For this review, take the finished solid that the model builds, in its own axes (mm). Face numbers are marked on the shaded views. A direction names the side the tool comes from. Give positions to 0.01 mm unless a question says otherwise; leave off trailing zeros. Write each loop counter-clockwise with the first axis right and the second up, starting at its lowest first coordinate (ties: lowest second). Pieces come first, ordered by that corner, then holes. Notation, with made-up numbers: M -3.75,-24.75 L 4.25,-24.75 A14 ccw 4.25,-8.75 Z; hole C -36.75,84 d11. An arc over 180 degrees is marked long. Answer as a JSON object with one key per item and string values. Group by question number.
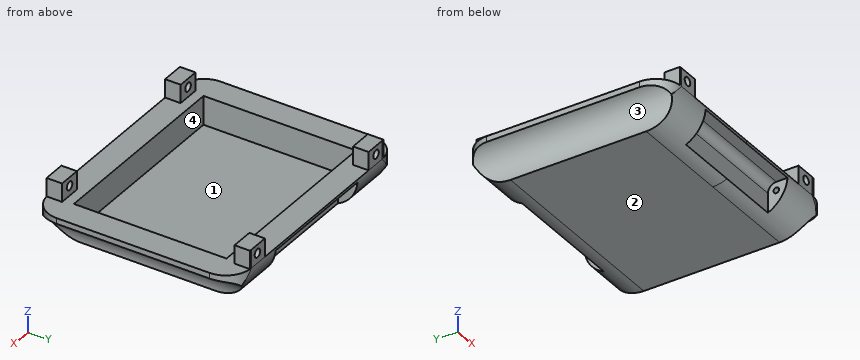
```python
from build123d import *

# Parameters (mm, degrees)
PAD003_DEPTH               = 18
POCKET008_DEPTH            = 22.126
POCKET008_DEPTH_BACK       = 22.126
SKETCH014_W                = 27
SKETCH014_H                = 5.1
POCKET009_DEPTH            = 17.5
POCKET010_DEPTH            = 11.05
SKETCH016_R                = 0.5
POCKET011_DEPTH            = 13.5
SKETCH018_W                = 4
SKETCH018_H                = 3.25
SKETCH018_R                = 0.75
PAD004_DEPTH               = 2.75
SKETCH018_MIRRORED005_2_W  = 4
SKETCH018_MIRRORED005_2_H  = 3.25
SKETCH018_MIRRORED005_2_R  = 0.75
PAD004_MIRRORED005_2_DEPTH = 2.75
SKETCH010_W                = 70
SKETCH010_H                = 70
POCKET013_DEPTH            = 6.001
POCKET013_DEPTH_BACK       = 3.251


with BuildPart() as part:
    # Sketch009 → Pad003 (new body, symmetric)
    with BuildSketch(Plane.XZ):
        with BuildLine():
            Line((-22.125, 0), (22.125, 0))
            Line((22.125, 0), (22.125, -1))
            ThreePointArc((22.125, -1), (19.164351, -2.759027), (18, -6))
            Line((-18, -6), (18, -6))
            ThreePointArc((-18, -6), (-19.164351, -2.759027), (-22.125, -1))
            Line((-22.125, 0), (-22.125, -1))
        make_face()
    extrude(amount=PAD003_DEPTH, both=True)

    # Sketch013 → Pocket008 (cut, two sides)
    with BuildSketch(Plane.YZ) as pocket008_sk:
        with BuildLine():
            ThreePointArc((-18, 0), (-16.242641, -4.242641), (-12, -6))
            Line((-12, -6), (-18, -6))
            Line((-18, 0), (-18, -6))
        make_face()
        with BuildLine():
            ThreePointArc((12, -6), (16.242641, -4.242641), (18, 0))
            Line((18, 0), (18, -6))
            Line((12, -6), (18, -6))
        make_face()
    extrude(amount=-POCKET008_DEPTH, mode=Mode.SUBTRACT)
    extrude(pocket008_sk.sketch, amount=POCKET008_DEPTH_BACK, mode=Mode.SUBTRACT)

    # Sketch014 → Pocket009 (cut, symmetric)
    with BuildSketch(Plane.YZ):
        with Locations((0, -2.55)):
            Rectangle(SKETCH014_W, SKETCH014_H)
    pocket009 = extrude(amount=POCKET009_DEPTH, both=True, mode=Mode.SUBTRACT)

    # Sketch015 → Pocket010 (cut, symmetric)
    with BuildSketch(Plane.YZ):
        with BuildLine():
            Line((16, -0.5), (18, -0.5))
            Line((18, -0.5), (18, -6))
            Line((18, -6), (14.5, -6))
            Line((14.5, -6), (14.5, -2))
            ThreePointArc((16, -0.5), (14.93934, -0.93934), (14.5, -2))
        make_face()
    pocket010 = extrude(amount=POCKET010_DEPTH, both=True, mode=Mode.SUBTRACT)

    # Sketch016 → Pocket011 (cut, symmetric)
    with BuildSketch(Plane.YZ):
        with Locations((16, -2)):
            Circle(SKETCH016_R)
    pocket011 = extrude(amount=POCKET011_DEPTH, both=True, mode=Mode.SUBTRACT)

    # Mirrored004: Pocket009, Pocket010, Pocket011 across Sketch014 V_Axis
    add(pocket009.mirror(Plane(origin=(0, 0, 0), x_dir=(1, 0, 0), z_dir=(0, 1, 0))), mode=Mode.SUBTRACT)
    add(pocket010.mirror(Plane(origin=(0, 0, 0), x_dir=(1, 0, 0), z_dir=(0, 1, 0))), mode=Mode.SUBTRACT)
    add(pocket011.mirror(Plane(origin=(0, 0, 0), x_dir=(1, 0, 0), z_dir=(0, 1, 0))), mode=Mode.SUBTRACT)

    # Sketch018 → Pad004 (join)
    with BuildSketch(Plane.XZ.offset(-18)):
        with Locations((16, 1.625)):
            Rectangle(SKETCH018_W, SKETCH018_H)
        with Locations((16, 1.75)):
            Circle(SKETCH018_R, mode=Mode.SUBTRACT)
    pad004 = extrude(amount=PAD004_DEPTH)

    # Sketch018 Mirrored005 2 → Pad004 Mirrored005 2 (add)
    with BuildSketch(Plane(origin=(0, 18, 0), x_dir=(-1, 0, 0), z_dir=(0, 1, 0))):
        with Locations((16, 1.625)):
            Rectangle(SKETCH018_MIRRORED005_2_W, SKETCH018_MIRRORED005_2_H)
        with Locations((16, 1.75)):
            Circle(SKETCH018_MIRRORED005_2_R, mode=Mode.SUBTRACT)
    pad004_mirrored005_2 = extrude(amount=-PAD004_MIRRORED005_2_DEPTH)

    # Mirrored006: Pad004, Pad004 Mirrored005 2 across XZ
    add(pad004.mirror(Plane.XZ))
    add(pad004_mirrored005_2.mirror(Plane.XZ))

    # Sketch010 → Pocket013 (cut, two sides)
    with BuildSketch(Plane.XY) as pocket013_sk:
        Rectangle(SKETCH010_W, SKETCH010_H)
        with BuildLine():
            ThreePointArc((-17.625, 18), (-20.806981, 16.681981), (-22.125, 13.5))
            Line((-22.125, 13.5), (-22.125, -13.5))
            ThreePointArc((-22.125, -13.5), (-20.806981, -16.681981), (-17.625, -18))
            Line((-17.625, -18), (17.625, -18))
            ThreePointArc((17.625, -18), (20.806981, -16.681981), (22.125, -13.5))
            Line((22.125, 13.5), (22.125, -13.5))
            ThreePointArc((22.125, 13.5), (20.806981, 16.681981), (17.625, 18))
            Line((17.625, 18), (-17.625, 18))
        make_face(mode=Mode.SUBTRACT)
    extrude(amount=-POCKET013_DEPTH, mode=Mode.SUBTRACT)
    extrude(pocket013_sk.sketch, amount=POCKET013_DEPTH_BACK, mode=Mode.SUBTRACT)


solid = part.part
```
Item 1: Insertion check: P1, Ø3, axis at x = -3, z = -3.5, coming from the -Y side; P2, Ø0.8, axis at y = 16, z = -2, coming from the -X side; P3, Ø5, axis at x = 4, y = -12.5, coming from the +Z side. Each pin has a flat end and moves straight along its axis. Give the tip position at first contact, or say it passes through.
Item 2: To check wall thickness, follow probe 1 along Y at (x, z) = (-3.5, -2); probe 2 along Z at (x, y) = (16, 4); probe 3 along X at (y, z) = (6, -1.75). State the ranges of each line that lie inside material, in increasing order.
Item 3: Consider section A-A (x = 16). Give the boundary of the cut face in (y, z).
Item 4: Consider section B-B (y = 10). Give the boundary of the cut face in (x, z) (3 decimals), plus the area to 3 significant figures.
Item 5: Draft analysis for pull direction Y (two halves, no side actions). For the marked faces 1 and 2, state which applies: released by +Y, released by -Y, zero draft, split by the parting line, or undercut.
Item 6: Machinability: for the marked faces 3 and 4, which of the approach directions +Z, -Z, +X, -X, +Y, -Y give a long, thin tool a straight path to every point of the face, cutting with its end or side? Answer none if there is none.
Item 7: Consider section C-C (x = 5.5). Give the boundary of the cut face in (y, z), plus the area to 3 significant figures.
Item 8: Consider section D-D (z = 1.75). State how many separate pieces and enclosed holes the cut face has, plus the area to 3 significant figures.
Result set:
{
 "1": {"P1": "stops at y = -14.5", "P2": "stops at x = -20.53", "P3": "stops at z = 0"},
 "2": {"probe 1": "y = -14.5 to -13.5, 13.5 to 14.5", "probe 2": "z = -6 to -5.1", "probe 3": "x = -20.29 to -17.5, 17.5 to 20.29"},
 "3": {"outline": "M -18,0 A6 ccw -12,-6 L 12,-6 A6 ccw 18,0 L 18,1 L 15.25,1 L 15.25,0 L 13.5,0 L 13.5,-5.1 L -13.5,-5.1 L -13.5,0 L -15.25,0 L -15.25,1 L -18,1 Z; M -18,2.5 L -15.25,2.5 L -15.25,3.25 L -18,3.25 Z; M 15.25,2.5 L 18,2.5 L 18,3.25 L 15.25,3.25 Z"},
 "4": {"outline": "M -22.125,-1 A5.093 cw -18,-6 L 18,-6 A5.093 cw 22.125,-1 L 22.125,0 L 17.5,0 L 17.5,-5.1 L -17.5,-5.1 L -17.5,0 L -22.125,0 Z", "area": "56.1 mm^2"},
 "5": {"face 1": "undercut", "face 2": "zero draft"},
 "6": {"face 3": "-Z, -X, +Y, -Y", "face 4": "+Z"},
 "7": {"outline": "M -18,0 A6 ccw -17.98,-0.5 L -16,-0.5 A1.5 cw -14.5,-2 L -14.5,-5.45 A6 ccw -12,-6 L 12,-6 A6 ccw 14.5,-5.45 L 14.5,-2 A1.5 cw 16,-0.5 L 17.98,-0.5 A6 ccw 18,0 L 13.5,0 L 13.5,-5.1 L -13.5,-5.1 L -13.5,0 Z", "area": "39.9 mm^2"},
 "8": {"separate pieces": "8", "enclosed holes": "0", "area": "27.5 mm^2"}
}
